Design review of the part built by this model. Coordinates are the model's own, in mm. Face numbers are marked on the shaded views. A direction names the side the tool comes from. Coordinates: 2 decimals unless noted, no trailing zeros. Write each loop counter-clockwise with the first axis right and the second up, starting at its lowest first coordinate (ties: lowest second). Pieces come first, ordered by that corner, then holes. Notation, with made-up numbers: (-37.5, -12) -> (13.5, -12) arc R23 cw to (13.5, 9) -> close; hole circle Ø8 at (39.25, 19.25). An arc over 180 degrees is marked (long way). Answer in a Markdown table with one row per item. Add a question column.
Item 1: Take a section at A-A, the plane z = -173. Write out the cut boundary in (x, y).
Item 2: Take a section at B-B, the plane y = 13. Write out the cut boundary in (x, z), and give its area (3 significant figures).
Item 3: To check wall thickness, follow line 1 (Y direction, x = 62, z = -29.5); line 2 (Z direction, x = 131.5, y = -260.5); line 3 (X direction, y = -269, z = 192). State the ranges of each line that lie inside material, in increasing order.
Item 4: For the marked faces 1 and 2, list the 3-axis set-ups (+Z, -Z, +X, -X, +Y, -Y) from which the entire face can be reached by the end or side of a thin tool; tool diameter is ignored.
Item 5: Clearance check with flat-ended pins moving along their axes: P1, Ø12, axis at y = 101.5, z = -166.5, coming from the -X side; P2, Ø1.5, axis at x = 42, y = 216, coming from the -Z side; P3, Ø4, axis at x = 172.5, y = 194.5, coming from the +Z side. State where each tip first meets the part, or that it passes through.
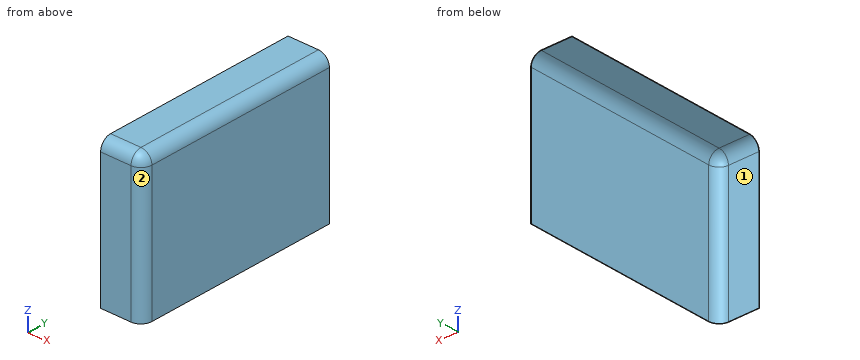
from build123d import *

# Parameters (mm, degrees)
F0_W     = 1000
F0_H     = 700
F1_DEPTH = 200
F2_W     = 997
F2_H     = 697
F3_DEPTH = 197
F4_R     = 50
F5_R     = 50
F6_R     = 53
F7_R     = 53


with BuildPart() as f1:
    # F0 (on Right) → F1 (new body)
    with BuildSketch(Plane.YZ):
        Rectangle(F0_W, F0_H)
    extrude(amount=F1_DEPTH)

    # F2 (on face) → F3 (cut)
    with BuildSketch(Plane(origin=(0, 0, 0), x_dir=(0, -1, 0), z_dir=(-1, 0, 0))):
        with Locations((-1.5, -1.5)):
            Rectangle(F2_W, F2_H)
    extrude(amount=-F3_DEPTH, mode=Mode.SUBTRACT)

    # F4
    f4_edges = [f1.edges().sort_by_distance(p)[0] for p in [
        (197, 1.5, 347),
    ]]
    fillet(f4_edges, radius=F4_R)

    # F5
    f5_edges = [f1.edges().sort_by_distance(p)[0] for p in [
        (197, -497, -26.5),
    ]]
    fillet(f5_edges, radius=F5_R)

    # F6
    f6_edges = [f1.edges().sort_by_distance(p)[0] for p in [
        (200, 0, 350),
    ]]
    fillet(f6_edges, radius=F6_R)

    # F7
    f7_edges = [f1.edges().sort_by_distance(p)[0] for p in [
        (200, -500, -26.5),
    ]]
    fillet(f7_edges, radius=F7_R)


solid = f1.part
Answers:
| question | item | result |
|---|---|---|
| 1 | outline | (0, -500) -> (147, -500) arc R53 ccw to (200, -447) -> (200, 500) -> (197, 500) -> (197, -447) arc R50 cw to (147, -497) -> (0, -497) -> close |
| 2 | outline | (0, 347) -> (147, 347) arc R50 cw to (197, 297) -> (197, -350) -> (200, -350) -> (200, 297) arc R53 ccw to (147, 350) -> (0, 350) -> close |
| 2 | area | 2,620 mm^2 |
| 3 | line 1 | y = -500 to -497 |
| 3 | line 2 | z = 347 to 350 |
| 3 | line 3 | x = 197 to 200 |
| 4 | face 1 | -Z, -X, +Y |
| 4 | face 2 | +Z, -Z, +X, -Y |
| 5 | P1 | stops at x = 197 |
| 5 | P2 | stops at z = 347 |
| 5 | P3 | stops at z = 344.51 |
